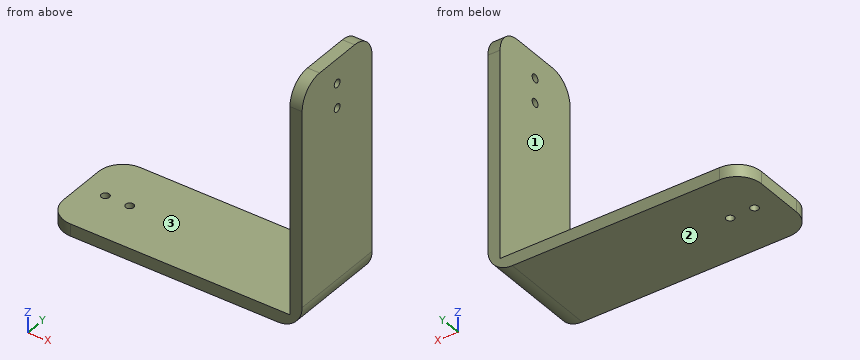
from build123d import *

# Parameters (mm, degrees)
EXTRUSION1_DEPTH   = 1
EXTRUSION3_DEPTH   = 1
D_GAGEMENT_00001_D = 0.6604
D_GAGEMENT_00002_D = 0.6604
D_GAGEMENT_00004_D = 0.6604
D_GAGEMENT_00005_D = 0.6604
CONG_2_R           = 2


with BuildPart() as part:
    # Esquisse1 → Extrusion1 (new body)
    with BuildSketch(Plane.XY):
        with BuildLine():
            Line((-52.829500905, 27.414750453), (-34.829500905, 27.414750453))
            Line((-34.829500905, 27.414750453), (-34.829500905, 19.414750453))
            Line((-34.829500905, 19.414750453), (-52.829500905, 19.414750453))
            ThreePointArc((-52.829500905, 19.414750453), (-54.243714467, 20.00053689), (-54.829500905, 21.414750453))
            Line((-54.829500905, 21.414750453), (-54.829500905, 25.414750453))
            ThreePointArc((-54.829500905, 25.414750453), (-54.243714467, 26.828964015), (-52.829500905, 27.414750453))
        make_face()
    extrude(amount=-EXTRUSION1_DEPTH)

    # Esquisse4 → Extrusion3 (add)
    with BuildSketch(Plane(origin=(-34.829500905, 0, 0), x_dir=(0, 0, -1), z_dir=(1, 0, 0))):
        with BuildLine():
            Line((1, 27.414750453), (-17, 27.414750453))
            ThreePointArc((-17, 27.414750453), (-18.414213562, 26.828964015), (-19, 25.414750453))
            Line((-19, 25.414750453), (-19, 21.414750453))
            ThreePointArc((-19, 21.414750453), (-18.414213562, 20.00053689), (-17, 19.414750453))
            Line((-17, 19.414750453), (1, 19.414750453))
            Line((1, 19.414750453), (1, 27.414750453))
        make_face()
    extrude(amount=EXTRUSION3_DEPTH)

    # Dégagement #00001 (through all)
    with Locations(Plane(origin=(-52.829500905, 23.414750453, 0), x_dir=(1, 0, 0), z_dir=(0, 0, 1))):
        with Locations((0, 0)):
            Hole(D_GAGEMENT_00001_D / 2)

    # Dégagement #00002 (through all)
    with Locations(Plane(origin=(-50.829500905, 23.414750453, 0), x_dir=(1, 0, 0), z_dir=(0, 0, 1))):
        with Locations((0, 0)):
            Hole(D_GAGEMENT_00002_D / 2)

    # Dégagement #00004 (through all)
    with Locations(Plane(origin=(-33.829500905, 23.414750453, 17), x_dir=(0, 0, 1), z_dir=(1, 0, 0))):
        with Locations((0, 0)):
            Hole(D_GAGEMENT_00004_D / 2)

    # Dégagement #00005 (through all)
    with Locations(Plane(origin=(-33.829500905, 23.414750453, 15), x_dir=(0, 0, 1), z_dir=(1, 0, 0))):
        with Locations((0, 0)):
            Hole(D_GAGEMENT_00005_D / 2)

    # Congé2
    cong_2_edges = [part.edges().sort_by_distance(p)[0] for p in [
        (-33.829500905, 23.414750453, -1),
    ]]
    fillet(cong_2_edges, radius=CONG_2_R)


solid = part.part
Verification items for the finished model (mm, model axes). Face numbers are marked on the shaded views. Give positions to 0.01 mm unless a question says otherwise; leave off trailing zeros. Order: outer loops, then holes, each group sorted by start corner. A loop starts at its lowest first (then second) coordinate and runs counter-clockwise, first axis right, second up. Notation, with made-up numbers: M -25.5,-28 L 2.5,-28 A28 ccw 2.5,8 Z; hole C 57.25,42 d1. An arc over 180 degrees is marked long. Use one line per item in the form item = value. Start each with the question number.
Q1. Scan lines: line 1 along Y through (x, z) = (-34.6, 15); line 2 along Z through (x, y) = (-47.75, 23); line 3 along X through (y, z) = (26.25, 4.75). Record each from-to range of solid material in increasing order. Write a range as [from, to].
Q2. Go/stop test with flat-tipped pins: pin 1 Ø4 at (x, y) = (-47, 23) entering from +Z; pin 2 Ø1 at (y, z) = (26, 12) entering from -X. Record where each tip stops, or that it passes through.
Q3. Section check C-C (x = -37.75). Enter the section's corners in (y, z), then the cut area to 3 significant figures.
Q4. Section check A-A (z = 15). Enter the section's corners in (x, y), then the cut area to 3 significant figures.
Q5. Mould release check, pull along Z, two halves, no side actions. Record for the marked faces 1, 2 and 3: +Z half, -Z half, draft (parallel to the pull), parting line (faces both ways), or undercut.
Q6. Section check D-D (z = 5). Enter the section's corners in (x, y).
Q7. Section check B-B (y = 22.75). Enter the section's corners in (x, z), then the cut area to 3 significant figures.
Evaluation:
q1.line_1 = [19.41, 23.08], [23.74, 27.41]
q1.line_2 = [-1, 0]
q1.line_3 = [-34.83, -33.83]
q2.pin_1 = 0
q2.pin_2 = -34.83
q3.outline = M 19.41,-1 L 27.41,-1 L 27.41,0 L 19.41,0 Z
q3.area = 8.00 mm2
q4.outline = M -34.83,19.41 L -33.83,19.41 L -33.83,23.08 L -34.83,23.08 Z; M -34.83,23.74 L -33.83,23.74 L -33.83,27.41 L -34.83,27.41 Z
q4.area = 7.34 mm2
q5.face_1 = draft
q5.face_2 = -Z half
q5.face_3 = +Z half
q6.outline = M -34.83,19.41 L -33.83,19.41 L -33.83,27.41 L -34.83,27.41 Z
q7.outline = M -54.83,-1 L -35.83,-1 A2 ccw -33.83,1 L -33.83,19 L -34.83,19 L -34.83,0 L -54.83,0 Z
q7.area = 39.1 mm2
